Could you check a few things on this model? Use its own coordinates, in mm. A direction names the side the tool comes from. Round coordinates to 2 decimals unless told otherwise and drop trailing zeros. Write each loop counter-clockwise with the first axis right and the second up, starting at its lowest first coordinate (ties: lowest second). Pieces come first, ordered by that corner, then holes. Notation, with made-up numbers: (79, 21.25) - (122, 21.25) arc R33 ccw to (122, 60.25) - close; hole circle Ø10 at (83.25, 21). An arc over 180 degrees is marked (long way). Write each question's results on one line, items separated by ' | '. Start each with the question number.
(1) Imagine slicing it at C-C on z = 12. Write out the boundary of the cut face in (x, y).
(2) On a 3-axis mill with a long thin cutter (end or side, diameter ignored), from which of +Z, -Z, +X, -X, +Y, -Y can I reach the whole of each face in a straight line? I mean faces 1 (the flat face through (0, -10, 6)), 2 (the flat face through (-5, 0, 5)), 3 (the flat face through (5, 0, 5)). Say none if no direction works.
(3) Imagine slicing it at B-B on x = -2.75. Write out the boundary of the cut face in (y, z), then the cut area to 3 significant figures.
(4) For P1, Ø5, axis at y = -0.5, z = 4, coming from the -X side; P2, Ø2, axis at x = 3, y = 0, coming from the +Z side; P3, Ø8, axis at y = 5.5, z = 2, coming from the +X side, each with a flat end and sliding along its axis, tell me the tip position at first contact or that it passes through.
(5) Please list where these lines run through material, in increasing order: line 1 (X direction, y = 5.5, z = 1.25); line 2 (X direction, y = 0.25, z = 13.5); line 3 (Z direction, x = -3, y = 6.75). Write a range as [from, to].
```python
from build123d import *

# Parameters (mm, degrees)
BOX001_W               = 7.1
BOX001_H               = 20
BOX001_DEPTH           = 7.1
BOX001_PLACEMENT_ANGLE = 45
BOX_W                  = 10
BOX_H                  = 20
BOX_DEPTH              = 10


with BuildPart() as obj1:
    # Box001 → Box001 (new body)
    with BuildSketch(Plane.XY):
        with Locations((3.55, 10)):
            Rectangle(BOX001_W, BOX001_H)
    extrude(amount=BOX001_DEPTH)


with BuildPart() as obj1_1:
    # Box001 placement: moved
    add(obj1.part.moved(Location((5, 0, 5))).rotate(Axis((5, 0, 5), (0, -1, 0)), BOX001_PLACEMENT_ANGLE))


with BuildPart() as fusion:
    # Box → Box (new body)
    with BuildSketch(Plane.XY):
        with Locations((5, 10)):
            Rectangle(BOX_W, BOX_H)
    extrude(amount=BOX_DEPTH)

    # Fusion: union obj1
    add(obj1_1.part)


with BuildPart() as fusion_1:
    # Fusion placement: moved
    add(fusion.part.moved(Location((-5, -10, 0))))


solid = fusion_1.part
```
Response:
1) outline: (-3.04, -10) - (3.04, -10) - (3.04, 10) - (-3.04, 10) - close
2) face 1: +Z, -Z, +X, -X, -Y | face 2: -Z, -X, +Y, -Y | face 3: -Z, +X, +Y, -Y
3) outline: (-10, 0) - (10, 0) - (10, 12.29) - (-10, 12.29) - close | area: 246 mm²
4) P1: x = -5 | P2: z = 13.04 | P3: x = 5
5) line 1: [-5, 5] | line 2: [-1.54, 1.54] | line 3: [0, 12.04]
